from build123d import *

# Parameters (mm, degrees)
F0_R     = 38.1
F1_DEPTH = 2438.4
F2_R     = 34.925
F3_DEPTH = 2438.401
F4_R     = 92.075
F5_DEPTH = 76.2


with BuildPart() as f1:
    # F0 (on Top) → F1 (new body)
    with BuildSketch(Plane.XY):
        Circle(F0_R)
    extrude(amount=F1_DEPTH)

    # F2 (on Top) → F3 (cut, through all)
    with BuildSketch(Plane.XY):
        Circle(F2_R)
    extrude(amount=F3_DEPTH, mode=Mode.SUBTRACT)

    # F4 (on Right) → F5 (cut, symmetric)
    with BuildSketch(Plane.YZ):
        Circle(F4_R)
    extrude(amount=F5_DEPTH, both=True, mode=Mode.SUBTRACT)


solid = f1.part
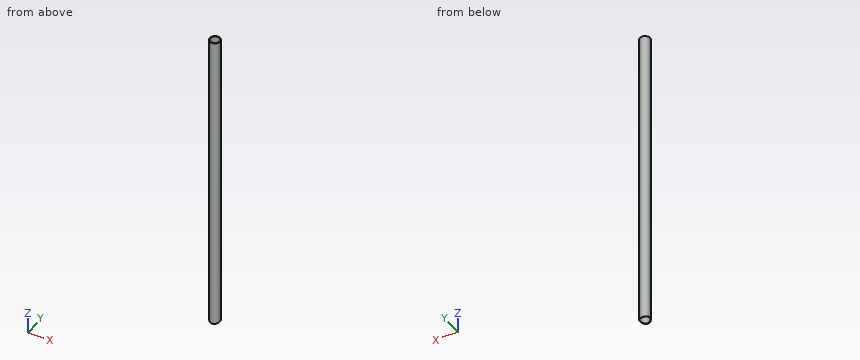
Model file for the job. Use its own axes, mm. Give positions to 0.01 mm unless a question says otherwise; leave off trailing zeros. Loops run counter-clockwise (first coordinate to the right, second up) from the corner with the lowest first, then second, coordinate; pieces in that order, holes last. Notation, with made-up numbers: (82.5, -24) -> (94.5, -24) arc R11 cw to (94.5, -18) -> close; hole circle Ø6 at (-8, 5). An arc over 180 degrees is marked (long way). Use a Markdown table: item, result. Add a question column.
(1) Wall check: line 1 along X through (y, z) = (0, 1710.5) (3 decimals); line 2 along Y through (x, z) = (29, 612). Give the ranges that are in metal, low to high.
(2) Drop flat-ended pins along their axis: pin 1 Ø4 at (y, z) = (-13.5, 1427.5) entering from +X; pin 2 Ø1.5 at (x, y) = (28, -24) entering from -Z; pin 3 Ø2 at (x, z) = (-24, 1575.5) entering from +Y. Give the stop position or say it passes through.
(3) Slice it at B-B on y = 18. List the corners of the cut face in (x, z), and give its area (3 significant figures).
(4) Slice it at A-A on x = 0. List the corners of the cut face in (y, z) (3 decimals).
Filled sheet:
| question | item | result |
|---|---|---|
| 1 | line 1 | -38.1 to -34.925, 34.925 to 38.1 |
| 1 | line 2 | -24.71 to -19.46, 19.46 to 24.71 |
| 2 | pin 1 | x = 36.32 |
| 2 | pin 2 | z = 88.69 |
| 2 | pin 3 | y = 30.37 |
| 3 | outline | (-33.58, 90.3) -> (-29.93, 90.3) -> (-29.93, 2438.4) -> (-33.58, 2438.4) -> close; (29.93, 90.3) -> (33.58, 90.3) -> (33.58, 2438.4) -> (29.93, 2438.4) -> close |
| 3 | area | 17,100 mm2 |
| 4 | outline | (-38.1, 83.822) arc R92.075 cw to (-34.925, 85.194) -> (-34.925, 2438.4) -> (-38.1, 2438.4) -> close; (34.925, 85.194) arc R92.075 cw to (38.1, 83.822) -> (38.1, 2438.4) -> (34.925, 2438.4) -> close |
